Read the model definition and answer for the solid it produces. Units are mm, in the model's axes. Face numbers are marked on the shaded views. Give positions to 0.01 mm unless a question says otherwise; leave off trailing zeros. Write each loop counter-clockwise with the first axis right and the second up, starting at its lowest first coordinate (ties: lowest second). Pieces come first, ordered by that corner, then holes.
```python
from build123d import *

# Parameters (mm, degrees)
BOSS_EXTRUDE1_DEPTH = 3.175


with BuildPart() as part:
    # Sketch1 → Boss-Extrude1 (new body)
    with BuildSketch(Plane.XY):
        with BuildLine():
            Line((-381, 3.615729939), (-381, 3.175))
            ThreePointArc((-381, 3.175), (-380.07006403, 0.92993597), (-377.825, 0))
            Line((-377.825, 0), (-342.9, 0))
            Line((-342.9, 0), (-342.9, 3.65125))
            ThreePointArc((-342.9, 3.65125), (-345.28125, 6.0325), (-342.9, 8.41375))
            Line((-342.9, 8.41375), (-342.9, 12.065))
            Line((-342.9, 12.065), (-378.295980938, 6.755602859))
            ThreePointArc((-378.295980938, 6.755602859), (-380.230825168, 5.68759631), (-381, 3.615729939))
        make_face()
        with BuildLine():
            Line((-342.9, 3.65125), (-342.9, 0))
            Line((-342.9, 0), (-336.55, 0))
            ThreePointArc((-336.55, 0), (-334.30493597, 0.92993597), (-333.375, 3.175))
            Line((-333.375, 3.175), (-333.375, 9.806979939))
            ThreePointArc((-333.375, 9.806979939), (-334.478133629, 12.212805107), (-337.020980938, 12.946852859))
            Line((-337.020980938, 12.946852859), (-342.9, 12.065))
            Line((-342.9, 12.065), (-342.9, 8.41375))
            ThreePointArc((-342.9, 8.41375), (-341.216201977, 7.716298023), (-340.51875, 6.0325))
            ThreePointArc((-340.51875, 6.0325), (-341.216201977, 4.348701977), (-342.9, 3.65125))
        make_face()
    extrude(amount=BOSS_EXTRUDE1_DEPTH)


solid = part.part
```
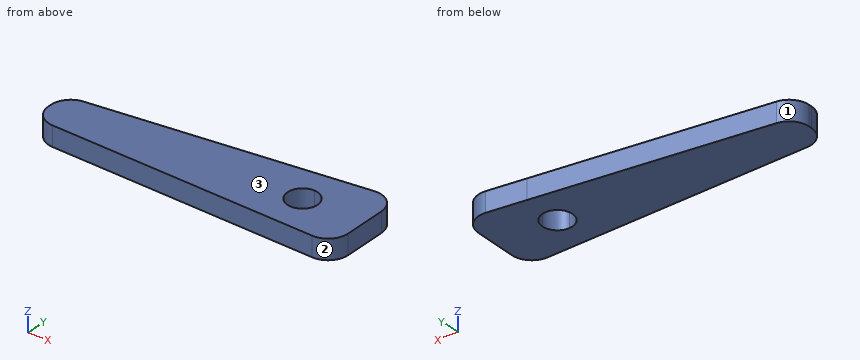
Item 1: Section C-C (y = 9.25) is taken. Write down the section's boundary in (x, z) (3 decimals).
Result set:
outline: (-361.667, 0) - (-333.375, 0) - (-333.375, 3.175) - (-361.667, 3.175) - close
Item 2: Section B-B (x = -360.5) is taken. Write down the section's boundary in (y, z) (3 decimals), and give its area (3 significant figures).
Result set:
outline: (0, 0) - (9.425, 0) - (9.425, 3.175) - (0, 3.175) - close
area: 29.9 mm2
Item 3: Determine the mould class of the marked faces 1, 2 and 3 for opening direction Y: pulls with the +Y half, pulls with the -Y half, needs draft (parallel to the pull), parting line crosses it, or undercut.
Result set:
face 1: pulls with the +Y half
face 2: pulls with the -Y half
face 3: needs draft
Item 4: Each of these flat-tipped pins is pushed along its axis until it touches: pin 1 Ø6 at (x, y) = (-356, 9.5) entering from -Z; pin 2 Ø1.5 at (x, z) = (-351, 2) entering from +Y. Where does it stop, or does it pass through?
Result set:
pin 1: stops at z = 0
pin 2: stops at y = 10.96
Item 5: Find the intervals of material crossed by line 1 along X through (y, z) = (4, 3) (3 decimals); line 2 along Y through (x, z) = (-341.5, 2.5) (3 decimals); line 3 along Y through (x, z) = (-341, 2.25), in increasing order.
Result set:
line 1: x = -380.977 to -344.141, -341.659 to -333.375
line 2: y = 0 to 4.106, 7.959 to 12.275
line 3: y = 0 to 4.6, 7.47 to 12.35
